from build123d import *

# Parameters (mm, degrees)
F1_DEPTH = 3
F2_W     = 42
F2_H     = 3
F2_W_2   = 8
F3_DEPTH = 25
F4_R     = 2
F5_DEPTH = 37.001
F6_R     = 1.5
F7_DEPTH = 37.001
F8_R     = 2
F9_DEPTH = 28.001


with BuildPart() as f1:
    # F0 (on Top) → F1 (new body)
    with BuildSketch(Plane.XY):
        Polygon((8, 8), (8, 0), (50, 0), (50, 8), (58, 8), (58, 34), (50, 34), (50, 37), (8, 37), (8, 34), (0, 34), (0, 8), align=None)
    extrude(amount=F1_DEPTH)

    # F2 (on face) → F3 (join)
    with BuildSketch(Plane.XY.offset(3)):
        with Locations((29, 1.5)):
            Rectangle(F2_W, F2_H)
        with Locations((4, 32.5)):
            Rectangle(F2_W_2, F2_H)
        with Locations((54, 32.5)):
            Rectangle(F2_W_2, F2_H)
    extrude(amount=F3_DEPTH)

    # F4 (on Front) → F5 (cut, through all)
    with BuildSketch(Plane.XZ):
        with Locations((54, 20)):
            Circle(F4_R)
        with Locations((54, 10)):
            Circle(F4_R)
        with Locations((4, 20)):
            Circle(F4_R)
        with Locations((4, 10)):
            Circle(F4_R)
    extrude(amount=-F5_DEPTH, mode=Mode.SUBTRACT)

    # F6 (on face) → F7 (cut, through all)
    with BuildSketch(Plane.XZ):
        with Locations((39.5, 14)):
            Circle(F6_R)
        with Locations((39.5, 21)):
            Circle(F6_R)
        with Locations((32.5, 14)):
            Circle(F6_R)
        with Locations((25.5, 14)):
            Circle(F6_R)
        with Locations((18.5, 14)):
            Circle(F6_R)
        with Locations((11.5, 14)):
            Circle(F6_R)
        with Locations((46.5, 14)):
            Circle(F6_R)
        with Locations((18.5, 21)):
            Circle(F6_R)
        with Locations((39.5, 7)):
            Circle(F6_R)
        with Locations((18.5, 7)):
            Circle(F6_R)
    extrude(amount=-F7_DEPTH, mode=Mode.SUBTRACT)

    # F8 (on face) → F9 (cut, through all)
    with BuildSketch(Plane(origin=(0, 0, 0), x_dir=(1, 0, 0), z_dir=(0, 0, -1))):
        with Locations((4, -15)):
            Circle(F8_R)
        with Locations((4, -25)):
            Circle(F8_R)
        with Locations((54, -25)):
            Circle(F8_R)
        with Locations((54, -15)):
            Circle(F8_R)
    extrude(amount=-F9_DEPTH, mode=Mode.SUBTRACT)


solid = f1.part
The model under review builds one solid part; all positions refer to its coordinate system, in mm. A direction names the side the tool comes from. Round coordinates to 2 decimals unless told otherwise and drop trailing zeros. Write each loop counter-clockwise with the first axis right and the second up, starting at its lowest first coordinate (ties: lowest second). Pieces come first, ordered by that corner, then holes. Notation, with made-up numbers: M 33.25,30.5 L 65.25,30.5 A29 ccw 65.25,54.5 Z; hole C 10,28 d4. An arc over 180 degrees is marked long. Use a Markdown table: item, result. Add a question column.
Q1. We need section C-C, the plane x = 54. State the section outline as (y, z) points, plus the area to 3 significant figures.
Q2. We need section D-D, the plane x = 32.5. State the section outline as (y, z) points, plus the area to 3 significant figures.
Q3. We need section A-A, the plane x = 39.5. State the section outline as (y, z) points, plus the area to 3 significant figures.
Q4. We need section B-B, the plane z = 7. State the section outline as (x, y) points.
Q5. The part is to be moulded in two halves that separate along Z. For faces 4 (the face through (4, 33, 28)), 5 (the face through (50, 35, 1)), 6 (the face through (54, 32, 22)), say which applies: pulls with the +Z half, pulls with the -Z half, needs draft (parallel to the pull), parting line crosses it, or undercut.
Q6. Machinability: for faces 1 (the face through (50, 2, 11)), 2 (the face through (4, 8, 1)), 3 (the face through (8, 32, 15)), which of the approach directions +Z, -Z, +X, -X, +Y, -Y give a long, thin tool a straight path to every point of the face, cutting with its end or side? Answer none if there is none.
Q7. To check wall thickness, follow line 1 (X direction, y = 25, z = 0.85); line 2 (Z direction, x = 18.5, y = 1.3); line 3 (Y direction, x = 44, z = 17). State the ranges of each line that lie inside material, in increasing order.
Q8. Insertion check: pin 1 (12 mm diameter, centred on y = 16.5, z = 9.5, fed in from -X); pin 2 (5 mm diameter, centred on x = 46.5, z = 14, fed in from +Y); pin 3 (0.9 mm diameter, centred on y = 35.5, z = 1.5, fed in from +X); pin 4 (1.5 mm diameter, centred on x = 34, y = 20, fed in from +Z). Each pin has a flat end and moves straight along its axis. Give the tip position at first contact, or say it passes through.
Findings below:
| question | item | result |
|---|---|---|
| 1 | outline | M 8,0 L 13,0 L 13,3 L 8,3 Z; M 17,0 L 23,0 L 23,3 L 17,3 Z; M 27,0 L 34,0 L 34,8 L 31,8 L 31,3 L 27,3 Z; M 31,12 L 34,12 L 34,18 L 31,18 Z; M 31,22 L 34,22 L 34,28 L 31,28 Z |
| 1 | area | 105 mm² |
| 2 | outline | M 0,0 L 37,0 L 37,3 L 3,3 L 3,12.5 L 0,12.5 Z; M 0,15.5 L 3,15.5 L 3,28 L 0,28 Z |
| 2 | area | 177 mm² |
| 3 | outline | M 0,0 L 37,0 L 37,3 L 3,3 L 3,5.5 L 0,5.5 Z; M 0,8.5 L 3,8.5 L 3,12.5 L 0,12.5 Z; M 0,15.5 L 3,15.5 L 3,19.5 L 0,19.5 Z; M 0,22.5 L 3,22.5 L 3,28 L 0,28 Z |
| 3 | area | 159 mm² |
| 4 | outline | M 0,31 L 8,31 L 8,34 L 0,34 Z; M 8,0 L 17,0 L 17,3 L 8,3 Z; M 20,0 L 38,0 L 38,3 L 20,3 Z; M 41,0 L 50,0 L 50,3 L 41,3 Z; M 50,31 L 58,31 L 58,34 L 50,34 Z |
| 5 | face 4 | pulls with the +Z half |
| 5 | face 5 | needs draft |
| 5 | face 6 | undercut |
| 6 | face 1 | +Z, -Z, +X, -Y |
| 6 | face 2 | +Z, -Z, -X, -Y |
| 6 | face 3 | +Z, +Y |
| 7 | line 1 | x = 0 to 2, 6 to 52, 56 to 58 |
| 7 | line 2 | z = 0 to 5.5, 8.5 to 12.5, 15.5 to 19.5, 22.5 to 28 |
| 7 | line 3 | y = 0 to 3 |
| 8 | pin 1 | passes through |
| 8 | pin 2 | stops at y = 3 |
| 8 | pin 3 | stops at x = 50 |
| 8 | pin 4 | stops at z = 3 |
